from build123d import *

# Parameters (mm, degrees)
ESBO_O1_W                = 49
ESBO_O1_H                = 45.64
RESSALTO_EXTRUS_O1_DEPTH = 31
CORTE_EXTRUS_O1_DEPTH    = 63.311735652
CORTE_EXTRUS_O2_DEPTH    = 63.311735652
ESBO_O5_R                = 1.35
CORTE_EXTRUS_O4_DEPTH    = 59.132775609
ESBO_O6_R                = 1.35
CORTE_EXTRUS_O5_DEPTH    = 44.646333179
FILETE1_R                = 2


with BuildPart() as part:
    # Esboço1 → Ressalto-extrusão1 (new body)
    with BuildSketch(Plane.XY):
        Rectangle(ESBO_O1_W, ESBO_O1_H)
    extrude(amount=RESSALTO_EXTRUS_O1_DEPTH)

    # Esboço2 → Corte-extrusão1 (cut, through all)
    with BuildSketch(Plane.ZY.offset(24.5)):
        Polygon((9.732649273, -22.82), (31, -22.82), (31, 14.022250108), align=None)
    extrude(amount=-CORTE_EXTRUS_O1_DEPTH, mode=Mode.SUBTRACT)

    # Esboço3 → Corte-extrusão2 (cut, through all)
    with BuildSketch(Plane.ZY.offset(24.5)):
        Polygon((0, -19.82), (8, -19.82), (28, 14.82), (28, 22.82), (0, 22.82), align=None)
    extrude(amount=-CORTE_EXTRUS_O2_DEPTH, mode=Mode.SUBTRACT)

    # Esboço5 → Corte-extrusão4 (cut, through all)
    with BuildSketch(Plane(origin=(0, -19.82, 0), x_dir=(1, 0, 0), z_dir=(0, 1, 0))):
        with Locations(Location((21.9, -2.6, 0), (0, 0, 180))):
            Circle(ESBO_O5_R)
        with Locations(Location((0, -2.6, 0), (0, 0, 180))):
            Circle(ESBO_O5_R)
        with Locations(Location((-21.9, -2.6, 0), (0, 0, 180))):
            Circle(ESBO_O5_R)
    extrude(amount=-CORTE_EXTRUS_O4_DEPTH, mode=Mode.SUBTRACT)

    # Esboço6 → Corte-extrusão5 (cut, through all)
    with BuildSketch(Plane(origin=(0, 0, 28), x_dir=(-1, 0, 0), z_dir=(0, 0, -1))):
        with Locations((21.9, 20.22)):
            Circle(ESBO_O6_R)
        with Locations((0, 20.22)):
            Circle(ESBO_O6_R)
        with Locations((-21.9, 20.22)):
            Circle(ESBO_O6_R)
    extrude(amount=-CORTE_EXTRUS_O5_DEPTH, mode=Mode.SUBTRACT)

    # Filete1
    filete1_edges = [part.edges().sort_by_distance(p)[0] for p in [
        (-24.5, -21.32, 0),
        (24.5, -21.32, 0),
        (-24.5, 22.82, 29.5),
        (24.5, 22.82, 29.5),
    ]]
    fillet(filete1_edges, radius=FILETE1_R)


solid = part.part
Part model, mm, in its own coordinate system. A direction names the side the tool comes from. Round coordinates to 2 decimals unless told otherwise and drop trailing zeros. Loops run counter-clockwise (first coordinate to the right, second up) from the corner with the lowest first, then second, coordinate; pieces in that order, holes last. Notation, with made-up numbers: (36.5, -7.75) - (85.5, -7.75) arc R14 ccw to (85.5, 18.25) - close; hole circle Ø2 at (75.5, 45.25). An arc over 180 degrees is marked (long way). Answer as a JSON object with one key per item and string values.
Item 1: Band-saw the part on D-D on x = 3.5. List the corners of the cut face in (y, z).
Output:
{"outline": "(-22.82, 0) - (-19.82, 0) - (-19.82, 8) - (14.82, 28) - (22.82, 28) - (22.82, 31) - (14.02, 31) - (-22.82, 9.73) - close"}
Item 2: Wall check: L1, parallel to X at y = 20, z = 29; L2, parallel to X at y = -20, z = 2; L3, parallel to Z at x = -9, y = 20.5. Give the ranges that are in metal, low to high.
Output:
{"L1": "-24.5 to -23.23, -20.57 to -1.33, 1.33 to 20.57, 23.23 to 24.5", "L2": "-24.5 to -23.11, -20.69 to -1.21, 1.21 to 20.69, 23.11 to 24.5", "L3": "28 to 31"}
Item 3: Pin check, flat tips, straight feed: pin 1 (3 mm diameter, centred on x = 0, y = 20.22, fed in from -Z); pin 2 (5 mm diameter, centred on x = -1, y = 6.5, fed in from -Z); pin 3 (1 mm diameter, centred on x = -11, z = 13.5, fed in from -Y); pin 4 (4.5 mm diameter, centred on x = -21.9, z = 2.6, fed in from -Y). Stop position of each tip, or through.
Output:
{"pin 1": "z = 28", "pin 2": "z = 21.75", "pin 3": "y = -17.16", "pin 4": "y = -22.82"}
Item 4: Band-saw the part on C-C on x = 21.9. List the corners of the cut face in (y, z).
Output:
{"outline": "(-22.82, 0) - (-19.82, 0) - (-19.82, 1.25) - (-22.82, 1.25) - close; (-22.82, 3.95) - (-19.82, 3.95) - (-19.82, 8) - (14.82, 28) - (18.87, 28) - (18.87, 31) - (14.02, 31) - (-22.82, 9.73) - close; (21.57, 28) - (22.82, 28) - (22.82, 31) - (21.57, 31) - close"}
Item 5: Pull direction X, two halves, no side cores. Call faces 1 (the face through (23.25, 20.28, 29.48)), 2 (the face through (23.9, 22.25, 29.52)), 3 (the face through (0, -19.82, 5)): pulls with the +X half, pulls with the -X half, needs draft (parallel to the pull), parting line crosses it, or undercut.
Output:
{"face 1": "undercut", "face 2": "pulls with the +X half", "face 3": "needs draft"}
Item 6: Band-saw the part on A-A on z = 2.6. List the corners of the cut face in (x, y).
Output:
{"outline": "(-24.5, -22.82) - (-23.25, -22.82) - (-23.25, -19.82) - (-24.5, -19.82) - close; (-20.55, -22.82) - (-1.35, -22.82) - (-1.35, -19.82) - (-20.55, -19.82) - close; (1.35, -22.82) - (20.55, -22.82) - (20.55, -19.82) - (1.35, -19.82) - close; (23.25, -22.82) - (24.5, -22.82) - (24.5, -19.82) - (23.25, -19.82) - close"}
Item 7: Tool access for faces 4 (the face through (-23.93, 22.22, 29.52)), 5 (the face through (0, 18, 28)): list every direction of +Z, -Z, +X, -X, +Y, -Y with a clear straight run to the whole face (end or side of a thin tool).
Output:
{"face 4": "+Z, -Z, -X, +Y", "face 5": "-Z, +X, -X, +Y"}
Item 8: Band-saw the part on B-B on y = 20.22. List the corners of the cut face in (x, z).
Output:
{"outline": "(-24.5, 28) - (-23.25, 28) - (-23.25, 31) - (-24.5, 31) - close; (-20.55, 28) - (-1.35, 28) - (-1.35, 31) - (-20.55, 31) - close; (1.35, 28) - (20.55, 28) - (20.55, 31) - (1.35, 31) - close; (23.25, 28) - (24.5, 28) - (24.5, 31) - (23.25, 31) - close"}
